Geometry check sheet. Reference: the model listing, model coordinates, mm. Face numbers are marked on the shaded views. A direction names the side the tool comes from. Coordinates: 2 decimals unless noted, no trailing zeros. Loops run counter-clockwise (first coordinate to the right, second up) from the corner with the lowest first, then second, coordinate; pieces in that order, holes last. Notation, with made-up numbers: M 67.25,-20 L 86.25,-20 A30 ccw 86.25,13 Z; hole C 36.25,18.25 d5. An arc over 180 degrees is marked long. One line per question, with ' | ' between items. Start each with the question number.
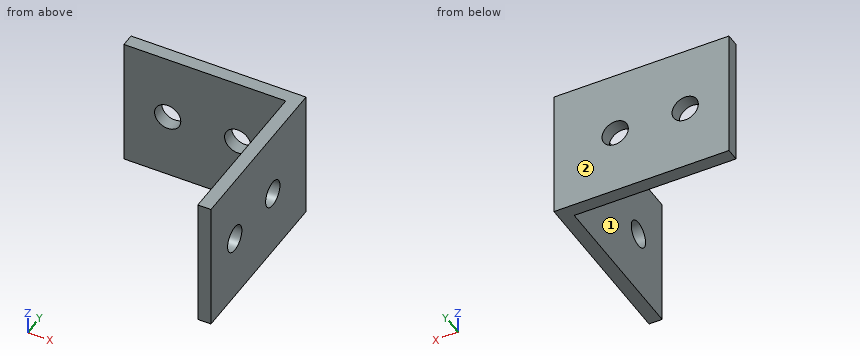
Autodesk Inventor part; units mm, degrees
ref_plane "YZ Plane" through (0, 0, 0) normal (1, 0, 0) x (0, 1, 0)
ref_plane "XZ Plane" through (0, 0, 0) normal (0, 1, 0) x (-1, 0, 0)
ref_plane "XY Plane" through (0, 0, 0) normal (0, 0, 1) x (1, 0, 0)
sketch "スケッチ1" plane through (0, 0, 0) normal (0, 1, 0) x (-1, 0, 0)
  line L0 (0, 0) -> (20, 0)
  line L1 (20, 0) -> (20, -15)
  line L2 (20, -15) -> (0, -15)
  line L3 (0, -15) -> (0, 0)
  dimension "d0" = 20
  dimension "d1" = 15
sketch "スケッチ2" plane through (0, 0, 0) normal (1, 0, 0) x (0, 1, 0)
  line L0 (0, 0) -> (-20, 0)
  line L1 (-20, 0) -> (-20, -15)
  line L2 (-20, -15) -> (0, -15)
  line L3 (0, -15) -> (0, 0)
  dimension "d2" = 20
  dimension "d3" = 15
extrude "押し出し1" add sketch "スケッチ1" along normal blind 1.5
extrude "押し出し2" add sketch "スケッチ2" along normal blind 1.5
sketch "スケッチ3" plane through (0, 0, 0) normal (0, 1, 0) x (1, 0, 0)
  line L0 (0, 15) -> (1.5, 15)
  line L1 (0, 0) -> (0, 15)
  line L2 (1.5, 15) -> (0, 15)
  line L3 (0, 15) -> (0, 0)
  line L4 (0, 0) -> (1.5, 0)
  line L5 (1.5, 0) -> (1.5, 15)
extrude "押し出し3" add sketch "スケッチ3" along normal blind 1.5
sketch "スケッチ4" plane through (1.5, 0, 0) normal (1, 0, 0) x (0, 0, -1)
  point P0 (0, 0)
sketch "スケッチ5" plane through (1.5, 0, 0) normal (1, 0, 0) x (0, 0, -1)
  point P0 (0, 0)
sketch "スケッチ6" plane through (-20, 0, -15) normal (-1, 0, 0) x (0, 0, 1)
  point P0 (15, 0)
sketch "スケッチ7" plane through (-20, 0, -15) normal (-1, 0, 0) x (0, 0, 1)
  line L0 (15.9074, 4.1741) -> (-1.7689, 4.1741)
  line L1 (-1.7689, 4.1741) -> (-1.7689, -3.4482)
  line L2 (-1.7689, -3.4482) -> (15.9074, -3.4482)
  line L3 (15.9074, -3.4482) -> (15.9074, 4.1741)
  point P0 (15, 0)
extrude "押し出し4" cut sketch "スケッチ7" against normal blind 1.5
sketch "スケッチ8" plane through (0, -20, -15) normal (0, -1, 0) x (1, 0, 0)
  line L0 (-2.0326, 16.6333) -> (6.4245, 16.6333)
  line L1 (6.4245, 16.6333) -> (6.4245, -1.5875)
  line L2 (6.4245, -1.5875) -> (-2.0326, -1.5875)
  line L3 (-2.0326, -1.5875) -> (-2.0326, 16.6333)
  point P0 (0, 15)
extrude "押し出し5" cut sketch "スケッチ8" against normal blind 1.5
sketch "スケッチ9" plane through (0, 1.5, 0) normal (0, 1, 0) x (1, 0, 0)
  circle A0 centre (-13.5, 7.5) radius 1.5
  circle A1 centre (-5.5, 7.5) radius 1.5
  point P0 (0, 0)
  dimension "d14" = 3
  dimension "d15" = 3
sketch "スケッチ10" plane through (1.5, 0, 0) normal (1, 0, 0) x (0, 0, -1)
  circle A0 centre (7.5, -5.5) radius 1.5
  circle A1 centre (7.5, -13.5) radius 1.5
  point P0 (0, 0)
  dimension "d16" = 3
  dimension "d18" = 3
extrude "押し出し6" cut sketch "スケッチ10" against normal blind 1.5
extrude "押し出し7" cut sketch "スケッチ9" against normal blind 1.5
properties part number "二つ分け角柱"
1. Sectioned sample at B-B (z = -7.5). Record the cut outline in (x, y).
2. Sectioned sample at D-D (z = -13.5). Record the cut outline in (x, y), and give its area (4 significant figures).
3. Sectioned sample at A-A (y = -5.5). Record the cut outline in (x, z), and give its area (3 significant figures).
4. Tool access check on the marked faces 1 and 2. Record the directions out of +Z, -Z, +X, -X, +Y, -Y that give a thin tool (end or side, any length) a straight path to the whole face; none if there is none.
5. Depth check by flat-ended pin: pin 1 Ø8 at (x, y) = (-0.5, -11.5) entering from -Z; pin 2 Ø2.5 at (x, z) = (-5.5, -7.5) entering from +Y; pin 3 Ø1.5 at (x, z) = (-13.5, -9.5) entering from -Y. Enter the tip coordinate at first touch or a pass-through.
6. Thickness scan on line 1 (X direction, y = 0.7, z = -7.5); line 2 (Z direction, x = -13.5, y = 0.55). Record the ranges inside material, lowest first.
Result:
1) outline: M -18.5,0 L -15,0 L -15,1.5 L -18.5,1.5 Z; M -12,0 L -7,0 L -7,1.5 L -12,1.5 Z; M -4,0 L 0,0 L 0,-4 L 1.5,-4 L 1.5,1.5 L -4,1.5 Z; M 0,-18.5 L 1.5,-18.5 L 1.5,-15 L 0,-15 Z; M 0,-12 L 1.5,-12 L 1.5,-7 L 0,-7 Z
2) outline: M -18.5,0 L 0,0 L 0,-18.5 L 1.5,-18.5 L 1.5,1.5 L -18.5,1.5 Z | area: 57.75 mm2
3) outline: M 0,-15 L 1.5,-15 L 1.5,-9 L 0,-9 Z; M 0,-6 L 1.5,-6 L 1.5,0 L 0,0 Z | area: 18.0 mm2
4) face 1: +Z, -Z, -X, -Y | face 2: +Z, -Z, +X, -X, +Y
5) pin 1: stops at z = -15 | pin 2: passes through | pin 3: stops at y = 0
6) line 1: x = -18.5 to -15, -12 to -7, -4 to 1.5 | line 2: z = -15 to -9, -6 to 0
